from build123d import *

# Parameters (mm, degrees)
F0_W     = 38.1
F0_H     = 31.75
F1_DEPTH = 25.4
F3_DEPTH = 25.4
F4_DEPTH = 25.4
F5_W     = 12.7
F5_H     = 6.35
F6_DEPTH = 25.401


# Not quite as in the source:
# - a feature names something its author has since deleted; it is built from what else it names


with BuildPart() as f1:
    # F0 (on Front) → F1 (new body)
    with BuildSketch(Plane.XZ):
        with Locations((19.05, 15.875)):
            Rectangle(F0_W, F0_H)
    extrude(amount=F1_DEPTH)

    # F0 (on Front) → F3 (join)
    with BuildSketch(Plane.XZ):
        with Locations((19.05, 15.875)):
            Rectangle(F0_W, F0_H)
    extrude(amount=F3_DEPTH)

    # F0 (on Front) → F4 (join)
    with BuildSketch(Plane.XZ):
        with Locations((19.05, 15.875)):
            Rectangle(F0_W, F0_H)
    extrude(amount=F4_DEPTH)

    # F5 (on face) → F6 (cut, through all)
    with BuildSketch(Plane.XZ.offset(25.4)):
        Polygon((0, 31.75), (0, 0), (12.7, 31.75), align=None)
        Polygon((38.1, 31.75), (25.4, 31.75), (38.1, 0), align=None)
        with Locations((19.05, 3.175)):
            Rectangle(F5_W, F5_H)
    extrude(amount=-F6_DEPTH, mode=Mode.SUBTRACT)


solid = f1.part
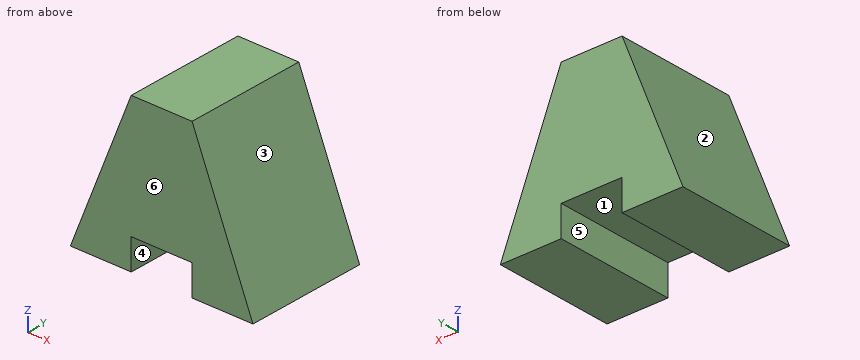
Can you work these out from the model? Positions are in its coordinate system, mm. Face numbers are marked on the shaded views. A direction names the side the tool comes from. Coordinates: 2 decimals unless noted, no trailing zeros. Loops run counter-clockwise (first coordinate to the right, second up) from the corner with the lowest first, then second, coordinate; pieces in that order, holes last. Notation, with made-up numbers: M -27.5,-17.75 L -21.5,-17.75 A21 ccw -21.5,9.25 Z; hole C 2,33.5 d7. An arc over 180 degrees is marked long. Answer as CSV lines item,"result". Start each with the question number.
1. Thinking about a two-plate mould opening in X: for the marked faces 3, 4, 5 and 6, which applies, +X half, -X half, draft (parallel to the pull), parting line (faces both ways), or undercut?
2. For the marked faces 1 and 2, which set-ups out of +Z, -Z, +X, -X, +Y, -Y let a thin tool reach every point of the face, with its end or its side?
3. For pin 1 Ø10 at (y, z) = (-18, 25) entering from +X; pin 2 Ø7 at (y, z) = (-11.5, 4.5) entering from -X; pin 3 Ø8 at (y, z) = (-15.5, 27) entering from +X, each with a flat end and sliding along its axis, tell me the tip position at first contact or that it passes through.
4. Suppose I cut it at B-B, the plane y = -23.5. List the corners of the cut face in (x, z) for me, plus the area to 3 significant figures.
5. If I drill on probe 1 along Z at (x, y) = (14.5, -5.5); probe 2 along X at (y, z) = (-9.5, 5.5); probe 3 along X at (y, z) = (-11.25, 4), over which ranges is the centre line in solid material (lowest first)? Write a range as [from, to].
6. Suppose I cut it at C-C, the plane x = 3. List the corners of the cut face in (y, z) for me, plus the area to 4 significant figures.
7. Suppose I cut it at D-D, the plane z = 21. List the corners of the cut face in (x, y) for me, plus the area to 3 significant figures.
8. Suppose I cut it at A-A, the plane z = 5.5. List the corners of the cut face in (x, y) for me.
Output:
1,face 3,"+X half"
1,face 4,"undercut"
1,face 5,"undercut"
1,face 6,"draft"
2,face 1,"-Z, +Y, -Y"
2,face 2,"+Z, -X, +Y, -Y"
3,pin 1,"stops at x = 30.1"
3,pin 2,"stops at x = 0.4"
3,pin 3,"stops at x = 28.9"
4,outline,"M 0,0 L 12.7,0 L 12.7,6.35 L 25.4,6.35 L 25.4,0 L 38.1,0 L 25.4,31.75 L 12.7,31.75 Z"
4,area,"726 mm^2"
5,probe 1,"z = [6.35, 31.75]"
5,probe 2,"x = [2.2, 12.7], [25.4, 35.9]"
5,probe 3,"x = [1.6, 12.7], [25.4, 36.5]"
6,outline,"M -25.4,0 L 0,0 L 0,7.5 L -25.4,7.5 Z"
6,area,"190.5 mm^2"
7,outline,"M 8.4,-25.4 L 29.7,-25.4 L 29.7,0 L 8.4,0 Z"
7,area,"541 mm^2"
8,outline,"M 2.2,-25.4 L 12.7,-25.4 L 12.7,0 L 2.2,0 Z; M 25.4,-25.4 L 35.9,-25.4 L 35.9,0 L 25.4,0 Z"
